Part print with two shaded views. Sizes in mm from the minimum x, y, z corner. Give positions to 0.01 mm unless a question says otherwise; leave off trailing zeros. Order: outer loops, then holes, each group sorted by start corner. A loop starts at its lowest first (then second) coordinate and runs counter-clockwise, first axis right, second up.
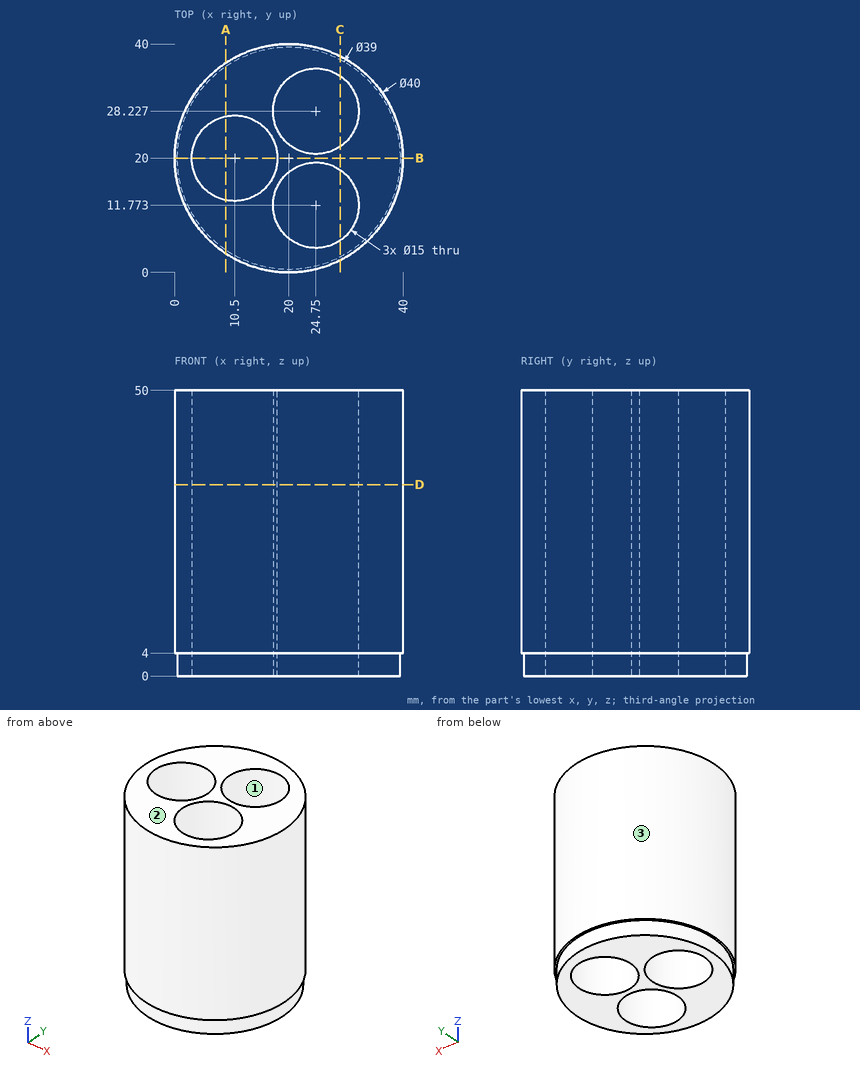
Item 1: Slice it at D-D (z = 33.5). Give the cut face in (x, y).
Item 2: Slice it at A-A (x = 9). Give the cut face in (y, z), and give its area (3 significant figures).
Item 3: Wall check: L1, parallel to X at y = 20, z = 5.5; L2, parallel to Y at x = 24, z = 18 (1 decimal); L3, parallel to Y at x = 24.75, z = 37.5. Give the ranges that are in metal, low to high.
Item 4: Two-plate mould, pull along Y, no slides. Class the marked faces 1, 2 and 3: released by +Y, released by -Y, zero draft, split by the parting line, or undercut.
Item 5: Slice it at B-B (y = 20). Give the cut face in (x, z), and give its area (3 significant figures).
Item 6: Slice it at C-C (x = 29). Give the cut face in (y, z).
Item 7: Drop flat-ended pins along their axis: pin 1 Ø10 at (x, z) = (15, 30.5) entering from -Y; pin 2 Ø5 at (y, z) = (14.5, 44) entering from -X; pin 3 Ø3 at (x, z) = (27, 31) entering from -Y. Give the stop position or say it passes through.
A:
1. outline: circle Ø40 at (20, 20); hole circle Ø15 at (10.5, 20); hole circle Ø15 at (24.75, 11.77); hole circle Ø15 at (24.75, 28.23)
2. outline: (3.3, 4) - (3.9, 4) - (3.9, 0) - (12.65, 0) - (12.65, 50) - (3.3, 50) - close; (27.35, 0) - (36.1, 0) - (36.1, 4) - (36.7, 4) - (36.7, 50) - (27.35, 50) - close
2. area: 931 mm2
3. L1: x = 0 to 3, 18 to 40
3. L2: y = 0.4 to 4.3, 19.2 to 20.8, 35.7 to 39.6
3. L3: y = 0.57 to 4.27, 19.27 to 20.73, 35.73 to 39.43
4. face 1: undercut
4. face 2: zero draft
4. face 3: split by the parting line
5. outline: (0, 4) - (0.5, 4) - (0.5, 0) - (3, 0) - (3, 50) - (0, 50) - close; (18, 0) - (39.5, 0) - (39.5, 4) - (40, 4) - (40, 50) - (18, 50) - close
5. area: 1,250 mm2
6. outline: (2.14, 4) - (2.7, 4) - (2.7, 0) - (5.59, 0) - (5.59, 50) - (2.14, 50) - close; (17.95, 0) - (22.05, 0) - (22.05, 50) - (17.95, 50) - close; (34.41, 0) - (37.3, 0) - (37.3, 4) - (37.86, 4) - (37.86, 50) - (34.41, 50) - close
7. pin 1: stops at y = 0
7. pin 2: stops at x = 0.23
7. pin 3: stops at y = 0.77
